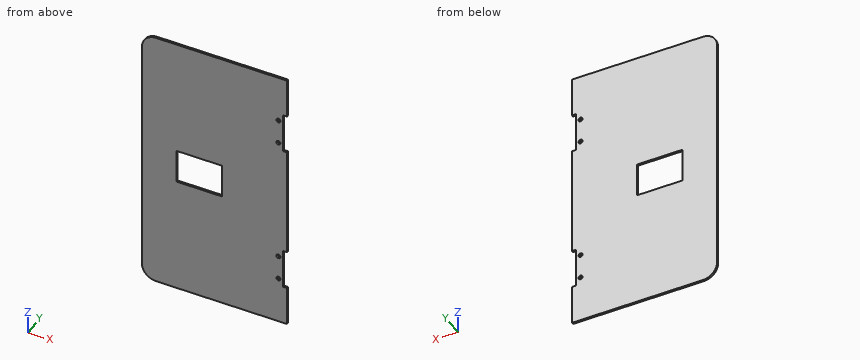
from build123d import *

# Parameters (mm, degrees)
F0_W     = 4
F0_H     = 42
F0_H_2   = 117
F1_DEPTH = 1
F2_R     = 15
F4_D     = 4.3
F4_DEPTH = 4
F4_TIP   = 1.2918503309
F5_W     = 48
F5_H     = 36
F6_DEPTH = 2


with BuildPart() as f1:
    # F0 (on Front) → F1 (new body, symmetric)
    with BuildSketch(Plane.XZ):
        Polygon((74, 100.5), (74, 142.5), (-74, 142.5), (-74, -142.5), (74, -142.5), (74, -100.5), (74, -58.5), (74, 58.5), align=None)
        with Locations((76, 121.5)):
            Rectangle(F0_W, F0_H)
        with Locations((76, 0)):
            Rectangle(F0_W, F0_H_2)
        with Locations((76, -121.5)):
            Rectangle(F0_W, F0_H)
    extrude(amount=F1_DEPTH, both=True)

    # F2
    f2_edges = [f1.edges().sort_by_distance(p)[0] for p in [
        (-74, 0, 142.5),
        (-74, 0, -142.5),
    ]]
    fillet(f2_edges, radius=F2_R)

    # F4
    with Locations(Plane(origin=(0, 1, 0), x_dir=(-1, 0, 0), z_dir=(0, 1, 0))):
        with Locations((-69, 92.5), (-69, 66.5), (-69, -92.5), (-69, -66.5)):
            Hole(F4_D / 2, depth=F4_DEPTH)
            with Locations((0, 0, -(F4_DEPTH + F4_TIP / 2))):  # 118° drill point
                Cone(0, F4_D / 2, F4_TIP, mode=Mode.SUBTRACT)

    # F5 (on face) → F6 (cut)
    with BuildSketch(Plane(origin=(0, 1, 0), x_dir=(-1, 0, 0), z_dir=(0, 1, 0))):
        with Locations((14, 0)):
            Rectangle(F5_W, F5_H)
    extrude(amount=-F6_DEPTH, mode=Mode.SUBTRACT)


solid = f1.part
Check sheet for the modelled part. Datum: model origin and axes. Units: mm. Round coordinates to 2 decimals unless told otherwise and drop trailing zeros. Order: outer loops, then holes, each group sorted by start corner. A loop starts at its lowest first (then second) coordinate and runs counter-clockwise, first axis right, second up.
(1) Cross-section at C-C, the plane y = -0.15. Enter the section's corners in (x, z), and give its area (3 significant figures).
(2) Scan lines: probe 1 along Z at (x, y) = (69, 0.35); probe 2 along Z at (x, y) = (6.5, 0.1); probe 3 along X at (y, z) = (-0.5, -17). Record each from-to range of solid material in increasing order.
(3) Go/stop test with a flat-tipped pin: P1, Ø2.5, axis at x = 69, z = -66.5, coming from the -Y side. Record where the tip stops, or that it passes through.
(4) Cross-section at B-B, the plane z = 1. Enter the section's corners in (x, y).
(5) Cross-section at A-A, the plane x = -31. Enter the section's corners in (y, z).
Check sheet entries:
1. outline: (-74, -127.5) arc R15 ccw to (-59, -142.5) - (78, -142.5) - (78, -100.5) - (74, -100.5) - (74, -58.5) - (78, -58.5) - (78, 58.5) - (74, 58.5) - (74, 100.5) - (78, 100.5) - (78, 142.5) - (-59, 142.5) arc R15 ccw to (-74, 127.5) - close; hole (-38, -18) - (10, -18) - (10, 18) - (-38, 18) - close; hole circle Ø4.3 at (69, -92.5); hole circle Ø4.3 at (69, -66.5); hole circle Ø4.3 at (69, 66.5); hole circle Ø4.3 at (69, 92.5)
1. area: 41,100 mm2
2. probe 1: z = -142.5 to -94.65, -90.35 to -68.65, -64.35 to 64.35, 68.65 to 90.35, 94.65 to 142.5
2. probe 2: z = -142.5 to -18, 18 to 142.5
2. probe 3: x = -74 to -38, 10 to 78
3. P1: passes through
4. outline: (-74, -1) - (-38, -1) - (-38, 1) - (-74, 1) - close; (10, -1) - (78, -1) - (78, 1) - (10, 1) - close
5. outline: (-1, -142.5) - (1, -142.5) - (1, -18) - (-1, -18) - close; (-1, 18) - (1, 18) - (1, 142.5) - (-1, 142.5) - close
